```python
from build123d import *

# Parameters (mm, degrees)
SKETCH1_R           = 49.276
BOSS_EXTRUDE1_DEPTH = 12.7
SKETCH1_10_R        = 28.952599956
CUT_EXTRUDE2_DEPTH  = 13.7
SKETCH2_R           = 12.7
CUT_EXTRUDE3_DEPTH  = 13.7


with BuildPart() as part:
    # Sketch1 → Boss-Extrude1 (new body)
    with BuildSketch(Plane(origin=(0, 0, 0), x_dir=(1, 0, 0), z_dir=(0, 1, 0))):
        Circle(SKETCH1_R)
    extrude(amount=BOSS_EXTRUDE1_DEPTH)

    # Sketch1<10> → Cut-Extrude2 (cut, through all)
    with BuildSketch(Plane(origin=(0, 0, 0), x_dir=(1, 0, 0), z_dir=(0, 1, 0))):
        Circle(SKETCH1_10_R)
    extrude(amount=CUT_EXTRUDE2_DEPTH, mode=Mode.SUBTRACT)

    # Sketch2 → Cut-Extrude3 (cut, through all)
    with BuildSketch(Plane(origin=(0, 12.7, 0), x_dir=(1, 0, 0), z_dir=(0, 1, 0))):
        with Locations((49.276, 0)):
            Circle(SKETCH2_R)
    extrude(amount=-CUT_EXTRUDE3_DEPTH, mode=Mode.SUBTRACT)


solid = part.part
```
The listing builds one solid part. Answer for the finished solid, in the listing's coordinates (mm). Coordinates: 2 decimals unless noted, no trailing zeros. Loops run counter-clockwise (first coordinate to the right, second up) from the corner with the lowest first, then second, coordinate; pieces in that order, holes last. Notation, with made-up numbers: (-5, 55.5) -> (39, 55.5) arc R34 ccw to (39, 93.5) -> close; hole circle Ø5 at (38, -33.75). An arc over 180 degrees is marked (long way). Use one line per item in the form item = value. Start each with the question number.
Item 1: The part is cut by section C-C on y = 10. Determine the outline of the cut face in (x, z).
Item 2: The part is cut by section B-B on z = 0. Determine the outline of the cut face in (x, y), then the cut area to 3 significant figures.
Item 3: The mould has two halves that part along X. Classify faces 1 (the face through (20, 12.7, 21.2)), 2 (the face through (-49.236, 6.261, -1.988)), 3 (the face through (-6.276, 6.261, 28.264)): released by +X, released by -X, zero draft, split by the parting line, or undercut.
Item 4: Flat-ended cylindrical pins translate along their axes: pin 1 Ø5 at (x, z) = (22.5, 11) entering from +Y; pin 2 Ø6 at (x, z) = (37.5, 1.5) entering from -Y; pin 3 Ø6 at (x, y) = (-13.5, 10) entering from -Z; pin 4 Ø6 at (y, z) = (3, 5.5) entering from -X. Find the tip coordinate at first contact, or state that the pin passes through.
Item 5: The part is cut by section D-D on z = 39. Determine the outline of the cut face in (x, y), then the cut area to 3 significant figures.
Item 6: Consider L1, parallel to X at y = 5.5, z = 0; L2, parallel to Z at x = 0, y = 3.5; L3, parallel to X at y = 7.25, z = -8. Determine where each line is inside the solid, lowest interval first. Write a range as [from, to].
Item 7: The part is cut by section A-A on x = 0. Determine the outline of the cut face in (y, z), then the cut area to 3 significant figures.
Answer key:
q1.outline = (47.64, -12.59) arc R12.7 cw to (47.64, 12.59) arc R49.28 ccw (long way) to start; hole circle Ø57.91 at (0, 0)
q2.outline = (-49.28, 0) -> (-28.95, 0) -> (-28.95, 12.7) -> (-49.28, 12.7) -> close; (28.95, 0) -> (36.58, 0) -> (36.58, 12.7) -> (28.95, 12.7) -> close
q2.area = 355 mm2
q3.face_1 = zero draft
q3.face_2 = split by the parting line
q3.face_3 = undercut
q4.pin_1 = through
q4.pin_2 = 0
q4.pin_3 = -48.14
q4.pin_4 = -49.21
q5.outline = (-30.12, 0) -> (30.12, 0) -> (30.12, 12.7) -> (-30.12, 12.7) -> close
q5.area = 765 mm2
q6.L1 = [-49.28, -28.95], [28.95, 36.58]
q6.L2 = [-49.28, -28.95], [28.95, 49.28]
q6.L3 = [-48.62, -27.83], [27.83, 39.41]
q7.outline = (0, -49.28) -> (12.7, -49.28) -> (12.7, -28.95) -> (0, -28.95) -> close; (0, 28.95) -> (12.7, 28.95) -> (12.7, 49.28) -> (0, 49.28) -> close
q7.area = 516 mm2
